```python
from build123d import *

# Parameters (mm, degrees)
SKETCH_1_W                = 6
SKETCH_1_H                = 38
EXTRUDE_1_DEPTH           = 8
HOLE_WIZARD_41_AT_2_COUNT = 2
HOLE_WIZARD_41_AT_2_PITCH = 22
CHAMFER_1_SIZE            = 0.449397949


with BuildPart() as part:
    # Эскиз1 → Бобышка-Вытянуть1 (new body)
    with BuildSketch(Plane.XY):
        Rectangle(SKETCH_1_W, SKETCH_1_H)
    extrude(amount=EXTRUDE_1_DEPTH)

    # Эскиз2 → Цековка для  винта с внутренним шестигранником #41 (revolve, cut)
    with BuildSketch(Plane(origin=(-0.5, 11, 0), x_dir=(0, 1, 0), z_dir=(1, 0, 0))):
        Polygon((0, 0), (0, 8), (1.6002, 8), (1.4732, 7.873), (1.4732, 2.9718), (1.6002, 2.8448), (2.77876, 2.8448), (2.77876, 0.127), (2.90576, 0), align=None)
    hole_wizard_41 = revolve(axis=Axis((-0.5, 11, -6.35), (0, 0, 1)), mode=Mode.SUBTRACT)

    # Цековка для  винта с внутренним шестигранником #41 at 2: Цековка для  винта с внутренним шестигранником #41 ×2
    with Locations(*[(0, -i * HOLE_WIZARD_41_AT_2_PITCH, 0) for i in range(1, HOLE_WIZARD_41_AT_2_COUNT)]):
        add(hole_wizard_41, mode=Mode.SUBTRACT)

    # Фаска1
    # the kernel refuses this chamfer: 0.5, 0.449397949 mm, written as the material it takes off along each edge
    with BuildSketch(Plane(origin=(-3, -9.786943061, 2.8448), x_dir=(0.5198491944846584, 0.8542580494169496, 0), z_dir=(0, 0, -1)), Plane(origin=(-3, 12.213056939, 2.8448), x_dir=(0.5198491944846584, 0.8542580494169496, 0), z_dir=(0, 0, -1))) as chamfer_1_piece_1:
        with BuildLine():
            Line((0.526718663, 0), (CHAMFER_1_SIZE * 0.854258048776, -CHAMFER_1_SIZE * 0.519849194094))
            Line((CHAMFER_1_SIZE * 0.854258048776, -CHAMFER_1_SIZE * 0.519849194094), (0, 0))
            ThreePointArc((0, 0), (0.268614935, -0.012503234), (0.526718663, 0))
        make_face()
    extrude(amount=4.061353185, mode=Mode.SUBTRACT)
    with BuildSketch(Plane(origin=(-3, -12.213056939, 2.8448), x_dir=(0.519849194484659, -0.8542580494169493, 0), z_dir=(0, 0, -1)), Plane(origin=(-3, 9.786943061, 2.8448), x_dir=(0.519849194484659, -0.8542580494169493, 0), z_dir=(0, 0, -1))) as chamfer_1_piece_2:
        with BuildLine():
            Line((0.526718663, 0), (CHAMFER_1_SIZE * 0.854258048776, CHAMFER_1_SIZE * 0.519849194094))
            Line((CHAMFER_1_SIZE * 0.854258048776, CHAMFER_1_SIZE * 0.519849194094), (0, 0))
            ThreePointArc((0, 0), (0.268614935, 0.012503234), (0.526718663, 0))
        make_face()
    extrude(amount=4.061353185, mode=Mode.SUBTRACT)


solid = part.part
```
CAD build for the part. Positions are in the model's coordinates, mm. A direction names the side the tool comes from. Coordinates: 2 decimals unless noted, no trailing zeros. Order: outer loops, then holes, each group sorted by start corner. A loop starts at its lowest first (then second) coordinate and runs counter-clockwise, first axis right, second up.
(1) Saw through at A-A, the plane y = -11. Write the cut outline in (x, z).
Solution:
outline: (-3, 2.84) - (-2.1, 2.84) - (-1.97, 2.97) - (-1.97, 7.87) - (-2.1, 8) - (-3, 8) - close; (0.97, 2.97) - (1.1, 2.84) - (2.28, 2.84) - (2.28, 0.13) - (2.41, 0) - (3, 0) - (3, 8) - (1.1, 8) - (0.97, 7.87) - close
(2) Saw through at D-D, the plane z = 1.5. Write the cut outline in (x, y), and give its area (3 significant figures).
Solution:
outline: (-3, -19) - (3, -19) - (3, 19) - (-3, 19) - (-3, 12.66) - (-2.73, 12.66) arc R2.78 cw (long way) to (-2.73, 9.34) - (-3, 9.34) - (-3, -9.34) - (-2.73, -9.34) arc R2.78 cw (long way) to (-2.73, -12.66) - (-3, -12.66) - close
area: 180 mm2
(3) Drill centre lines: L1, parallel to Y at x = -0.5, z = 0.8; L2, parallel to Y at x = -0.5, z = 4.15; L3, parallel to X at y = 11, z = 0.85. Where is each one in solid material? Low to high.
Solution:
L1: y = -19 to -13.78, -8.22 to 8.22, 13.78 to 19
L2: y = -19 to -12.47, -9.53 to 9.53, 12.47 to 19
L3: x = 2.28 to 3
(4) Saw through at C-C, the plane z = 5.5. Write the cut outline in (x, y).
Solution:
outline: (-3, -19) - (3, -19) - (3, 19) - (-3, 19) - close; hole circle Ø2.95 at (-0.5, -11); hole circle Ø2.95 at (-0.5, 11)
(5) Mould opens along Y. For faces 1 (the face through (0, 19, 4)), 2 (the face through (-0.56, -12.47, 5.39)), 3 (the face through (1, 12, 2.845)), 4 (the face through (0, 0, 8)) say: released by +Y, released by -Y, zero draft, split by the parting line, or undercut.
Solution:
face 1: released by +Y
face 2: undercut
face 3: undercut
face 4: zero draft
(6) Saw through at B-B, the plane x = -0.5. Count the separate pieces of the cut face and the enclosed holes in it, and give its area (3 significant figures).
Solution:
separate pieces: 3
enclosed holes: 0
area: 242 mm2
(7) Which spindle directions (+Z, -Z, +X, -X, +Y, -Y) get a long thin tool onto all of the face, cutting with end or side? Do faces 5 (the face through (2.277, 10.903, 1.467)), 6 (the face through (-3, 0, 4)). Say none if no direction does.
Solution:
face 5: -Z
face 6: +Z, -Z, -X, +Y, -Y
(8) Pin check, flat tip, straight feed: pin 1 Ø2.5 at (x, y) = (-0.5, -10.5) entering from -Z. Stop position of the tip, or through.
Solution:
pin 1: stops at z = 2.84
